Here's how the part is built. I have some questions about the finished solid (model axes, mm). Face numbers are marked on the shaded views. A direction names the side the tool comes from. Give positions to 0.01 mm unless a question says otherwise; leave off trailing zeros. Loops run counter-clockwise (first coordinate to the right, second up) from the corner with the lowest first, then second, coordinate; pieces in that order, holes last. Notation, with made-up numbers: (82, -39) -> (121, -39) arc R22 cw to (121, -18) -> close; hole circle Ø6 at (9.5, 3.25). An arc over 180 degrees is marked (long way). Answer in a Markdown table with one row per item. Add a question column.
Item 1: If we section it at A-A (z = 18): Write out the boundary of the cut face in (x, y).
Item 2: If we section it at B-B (y = 18.5): Write out the boundary of the cut face in (x, z).
Item 3: For P1, Ø5, axis at x = -46, z = 19.5, coming from the +Y side; P2, Ø2, axis at x = 15.5, z = 15, coming from the -Y side; P3, Ø1, axis at x = 6, z = 14.5, coming from the -Y side; P4, Ø21, axis at x = 32.04, y = -18.5, coming from the +Z side, each with a flat end and sliding along its axis, tell me the tip position at first contact or that it passes through.
Item 4: If I drill on line 1 (Y direction, x = 0, z = 5.25); line 2 (Z direction, x = 52.5, y = 0); line 3 (Y direction, x = 0, z = 18.5), over which ranges is the centre line in solid material (lowest first)?
Item 5: We'd pull the mould along X, two halves only. Please class the marked faces 3, 4 and 5: released by +X, released by -X, zero draft, split by the parting line, or undercut.
Item 6: If we section it at D-D (x = 33): Write out the boundary of the cut face in (y, z), then the cut area to 3 significant figures.
Item 7: Which directions (+Z, -Z, +X, -X, +Y, -Y) give clear straight access to the entire face, cutting with the end or side of a thin tool? Please do the marked faces 1 and 2.
Item 8: If we section it at C-C (x = -37.5): Write out the boundary of the cut face in (y, z), then the cut area to 3 significant figures.
```python
from build123d import *

# Parameters (mm, degrees)
SKETCH1_R              = 64
SKETCH1_R_2            = 60
RIM_DEPTH              = 28
SKETCH2_R              = 65.5
SKETCH2_R_2            = 63
INNER_BEAD_LIP_DEPTH   = 1.5
SKETCH3_R              = 65.5
SKETCH3_R_2            = 63
OUTER_BEAD_LIP_DEPTH   = 1.5
SKETCH4_R              = 61
WEB_DEPTH              = 7
SKETCH5_R              = 8
HUB_BOSS_DEPTH         = 24
SKETCH6_R              = 13
LIGHTENING_HOLES_DEPTH = 9
SKETCH7_R              = 3.15
ROUND_BORE_6MM_DEPTH   = 30
SKETCH8_R              = 1.3
GRUB_SCREW_M3_DEPTH    = 9
SKETCH9_R              = 1.9
GRUB_KEY_ACCESS_DEPTH  = 57.5


with BuildPart() as part:
    # Sketch1 → Rim (new body)
    with BuildSketch(Plane.XY):
        Circle(SKETCH1_R)
        Circle(SKETCH1_R_2, mode=Mode.SUBTRACT)
    extrude(amount=RIM_DEPTH)

    # Sketch2 → Inner_bead_lip (add)
    with BuildSketch(Plane.XY):
        Circle(SKETCH2_R)
        Circle(SKETCH2_R_2, mode=Mode.SUBTRACT)
    extrude(amount=INNER_BEAD_LIP_DEPTH)

    # Sketch3 → Outer_bead_lip (add)
    with BuildSketch(Plane.XY.offset(26.5)):
        Circle(SKETCH3_R)
        Circle(SKETCH3_R_2, mode=Mode.SUBTRACT)
    extrude(amount=OUTER_BEAD_LIP_DEPTH)

    # Sketch4 → Web (add)
    with BuildSketch(Plane.XY):
        Circle(SKETCH4_R)
    extrude(amount=WEB_DEPTH)

    # Sketch5 → Hub_boss (add)
    with BuildSketch(Plane.XY):
        Circle(SKETCH5_R)
    extrude(amount=HUB_BOSS_DEPTH)

    # Sketch6 → Lightening_holes (cut)
    with BuildSketch(Plane.XY.offset(-1)):
        with Locations((32.04293994, 18.5)):
            Circle(SKETCH6_R)
        with Locations((0, 37)):
            Circle(SKETCH6_R)
        with Locations((-32.04293994, 18.5)):
            Circle(SKETCH6_R)
        with Locations((-32.04293994, -18.5)):
            Circle(SKETCH6_R)
        with Locations((0, -37)):
            Circle(SKETCH6_R)
        with Locations((32.04293994, -18.5)):
            Circle(SKETCH6_R)
    extrude(amount=LIGHTENING_HOLES_DEPTH, mode=Mode.SUBTRACT)

    # Sketch7 → Round_bore_6mm (cut)
    with BuildSketch(Plane.XY.offset(-1)):
        Circle(SKETCH7_R)
    extrude(amount=ROUND_BORE_6MM_DEPTH, mode=Mode.SUBTRACT)

    # Sketch8 → Grub_screw_M3 (cut)
    with BuildSketch(Plane(origin=(0, 0, 0), x_dir=(0, 0, -1), z_dir=(1, 0, 0))):
        with Locations((-3.6, 0)):
            Circle(SKETCH8_R)
    extrude(amount=GRUB_SCREW_M3_DEPTH, mode=Mode.SUBTRACT)

    # Sketch9 → Grub_key_access (cut)
    with BuildSketch(Plane(origin=(8.5, 0, 0), x_dir=(0, 0, -1), z_dir=(1, 0, 0))):
        with Locations((-3.6, 0)):
            Circle(SKETCH9_R)
    extrude(amount=GRUB_KEY_ACCESS_DEPTH, mode=Mode.SUBTRACT)


solid = part.part
```
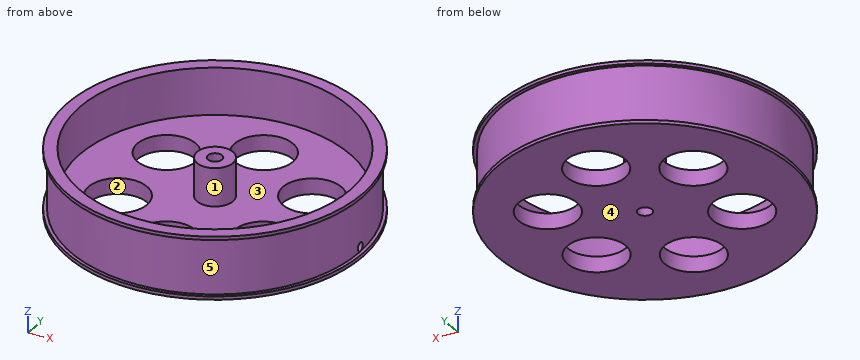
Recorded:
| question | item | result |
|---|---|---|
| 1 | outline | circle Ø128 at (0, 0); circle Ø16 at (0, 0); hole circle Ø120 at (0, 0); hole circle Ø6.3 at (0, 0) |
| 2 | outline | (-62.83, 0) -> (-45.04, 0) -> (-45.04, 7) -> (-57.08, 7) -> (-57.08, 28) -> (-62.83, 28) -> (-62.83, 26.5) -> (-61.27, 26.5) -> (-61.27, 1.5) -> (-62.83, 1.5) -> close; (-19.04, 0) -> (19.04, 0) -> (19.04, 7) -> (-19.04, 7) -> close; (45.04, 0) -> (62.83, 0) -> (62.83, 1.5) -> (61.27, 1.5) -> (61.27, 26.5) -> (62.83, 26.5) -> (62.83, 28) -> (57.08, 28) -> (57.08, 7) -> (45.04, 7) -> close |
| 3 | P1 | stops at y = 46.94 |
| 3 | P2 | stops at y = -62.34 |
| 3 | P3 | stops at y = -63.76 |
| 3 | P4 | passes through |
| 4 | line 1 | y = -64 to -50, -24 to -3.15, 3.15 to 24, 50 to 64 |
| 4 | line 2 | z = 0 to 1.7, 5.5 to 7 |
| 4 | line 3 | y = -64 to -60, -8 to -3.15, 3.15 to 8, 60 to 64 |
| 5 | face 3 | undercut |
| 5 | face 4 | zero draft |
| 5 | face 5 | split by the parting line |
| 6 | outline | (-56.58, 0) -> (-31.46, 0) -> (-31.46, 7) -> (-50.11, 7) -> (-50.11, 28) -> (-56.58, 28) -> (-56.58, 26.5) -> (-54.84, 26.5) -> (-54.84, 1.5) -> (-56.58, 1.5) -> close; (-5.54, 0) -> (5.54, 0) -> (5.54, 7) -> (-5.54, 7) -> close; (31.46, 0) -> (56.58, 0) -> (56.58, 1.5) -> (54.84, 1.5) -> (54.84, 26.5) -> (56.58, 26.5) -> (56.58, 28) -> (50.11, 28) -> (50.11, 7) -> (31.46, 7) -> close; hole circle Ø3.8 at (0, 3.6) |
| 6 | area | 602 mm^2 |
| 7 | face 1 | +Z |
| 7 | face 2 | +Z, -Z |
| 8 | outline | (-53.7, 0) -> (-30.3, 0) -> (-30.3, 7) -> (-46.84, 7) -> (-46.84, 28) -> (-53.7, 28) -> (-53.7, 26.5) -> (-51.86, 26.5) -> (-51.86, 1.5) -> (-53.7, 1.5) -> close; (-6.7, 0) -> (6.7, 0) -> (6.7, 7) -> (-6.7, 7) -> close; (30.3, 0) -> (53.7, 0) -> (53.7, 1.5) -> (51.86, 1.5) -> (51.86, 26.5) -> (53.7, 26.5) -> (53.7, 28) -> (46.84, 28) -> (46.84, 7) -> (30.3, 7) -> close |
| 8 | area | 618 mm^2 |
